Geometry check sheet. Reference: the model listing, model coordinates, mm. A direction names the side the tool comes from. Round coordinates to 2 decimals unless told otherwise and drop trailing zeros. Order: outer loops, then holes, each group sorted by start corner. A loop starts at its lowest first (then second) coordinate and runs counter-clockwise, first axis right, second up. Notation, with made-up numbers: (-36, 39.5) - (-28, 39.5) arc R7 cw to (-28, 43.5) - close; hole circle Ø9 at (70.5, 41.25). An arc over 180 degrees is marked (long way). Use a Markdown table: item, result. Add a question column.
(1) Gauge pin test, flat ends, axial feed: P1, Ø5, axis at x = 11.5, y = -1, coming from the -Z side; P2, Ø8, axis at x = 0, z = 0, coming from the -Y side; P3, Ø12, axis at y = -3, z = 1, coming from the -X side; P4, Ø5, axis at x = 3, z = 4, coming from the +Y side. Record the tip position at first contact, or that the pin passes through.
(2) Mould release check, pull along Z, two halves, no side actions. Record for faces 1 (the face through (3, -12, -10)), 2 (the face through (-14.985, -1.647, 0.66)), 3 (the face through (-2.17, 4.44, -9.76)): released by +Z, released by -Z, zero draft, split by the parting line, or undercut.
(3) Access from +Z, -Z, +X, -X, +Y, -Y to the whole of each face (thin tool, end or side, straight path). Record for faces 4 (the face through (2, -3, -2)), 5 (the face through (2, 0, -2)), 6 (the face through (3, 9, -10)).
(4) Thickness scan on line 1 along Z through (x, y) = (0, -0.7); line 2 along Y through (x, z) = (-3.75, 6.5); line 3 along Z through (x, y) = (1.5, -10). Record the ranges inside material, lowest first. Write a range as [from, to].
(5) Section check C-C on y = 5. Record the boundary of the cut face in (x, z), then the cut area to 3 significant figures.
(6) Section check D-D on x = -5.25. Record the boundary of the cut face in (y, z), then the cut area to 3 significant figures.
(7) Section check B-B on x = 0. Record the boundary of the cut face in (y, z), then the cut area to 3 significant figures.
(8) Section check A-A on z = 0. Record the boundary of the cut face in (x, y).
```python
from build123d import *

# Parameters (mm, degrees)
F0_R          = 15
F1_DEPTH      = 12
F1_DEPTH_BACK = 9
F3_D          = 20
F4_R          = 13.574911
F5_DEPTH      = 3
F7_D          = 5


with BuildPart() as f1:
    # F0 (on Front) → F1 (new body, two sides)
    with BuildSketch(Plane.XZ) as f1_sk:
        Circle(F0_R)
    extrude(amount=F1_DEPTH)
    extrude(f1_sk.sketch, amount=-F1_DEPTH_BACK)

    # F3 (through all)
    with Locations(Plane(origin=(0, 9, 0), x_dir=(-1, 0, 0), z_dir=(0, 1, 0))):
        with Locations((0, 0)):
            Hole(F3_D / 2)

    # F4 (on Front) → F5 (join)
    with BuildSketch(Plane.XZ):
        Circle(F4_R)
    extrude(amount=F5_DEPTH)

    # F7 (through all)
    with Locations(Plane.XZ.offset(3)):
        with Locations((0, 0)):
            Hole(F7_D / 2)


solid = f1.part
```
Check sheet entries:
| question | item | result |
|---|---|---|
| 1 | P1 | stops at z = -12 |
| 1 | P2 | stops at y = -3 |
| 1 | P3 | stops at x = -15 |
| 1 | P4 | stops at y = 0 |
| 2 | face 1 | zero draft |
| 2 | face 2 | split by the parting line |
| 2 | face 3 | undercut |
| 3 | face 4 | -Y |
| 3 | face 5 | +Y |
| 3 | face 6 | +Z, -Z, +X, -X, +Y |
| 4 | line 1 | z = [-15, -2.5], [2.5, 15] |
| 4 | line 2 | y = [-3, 0] |
| 4 | line 3 | z = [-14.92, -9.89], [9.89, 14.92] |
| 5 | outline | circle Ø30 at (0, 0); hole circle Ø20 at (0, 0) |
| 5 | area | 393 mm2 |
| 6 | outline | (-12, -14.05) - (9, -14.05) - (9, -8.51) - (0, -8.51) - (0, 8.51) - (9, 8.51) - (9, 14.05) - (-12, 14.05) - (-12, 8.51) - (-3, 8.51) - (-3, -8.51) - (-12, -8.51) - close |
| 6 | area | 284 mm2 |
| 7 | outline | (-12, -15) - (9, -15) - (9, -10) - (0, -10) - (0, -2.5) - (-3, -2.5) - (-3, -10) - (-12, -10) - close; (-12, 10) - (-3, 10) - (-3, 2.5) - (0, 2.5) - (0, 10) - (9, 10) - (9, 15) - (-12, 15) - close |
| 7 | area | 255 mm2 |
| 8 | outline | (-15, -12) - (-10, -12) - (-10, -3) - (-2.5, -3) - (-2.5, 0) - (-10, 0) - (-10, 9) - (-15, 9) - close; (2.5, -3) - (10, -3) - (10, -12) - (15, -12) - (15, 9) - (10, 9) - (10, 0) - (2.5, 0) - close |
